Answer from the drawing. Dimensions are ordinates in mm from the lowest x, y and z of the part. Give positions to 0.01 mm unless a question says otherwise; leave off trailing zeros. Order: outer loops, then holes, each group sorted by start corner. A loop starts at its lowest first (then second) coordinate and runs counter-clockwise, first axis right, second up. Notation, with made-up numbers: (34.25, 24.25) - (93.25, 24.25) arc R19 cw to (93.25, 60.25) - close; hole circle Ø7 at (61, 35). An arc over 180 degrees is marked (long way). Write each question's results on one line, items separated by ' | '.
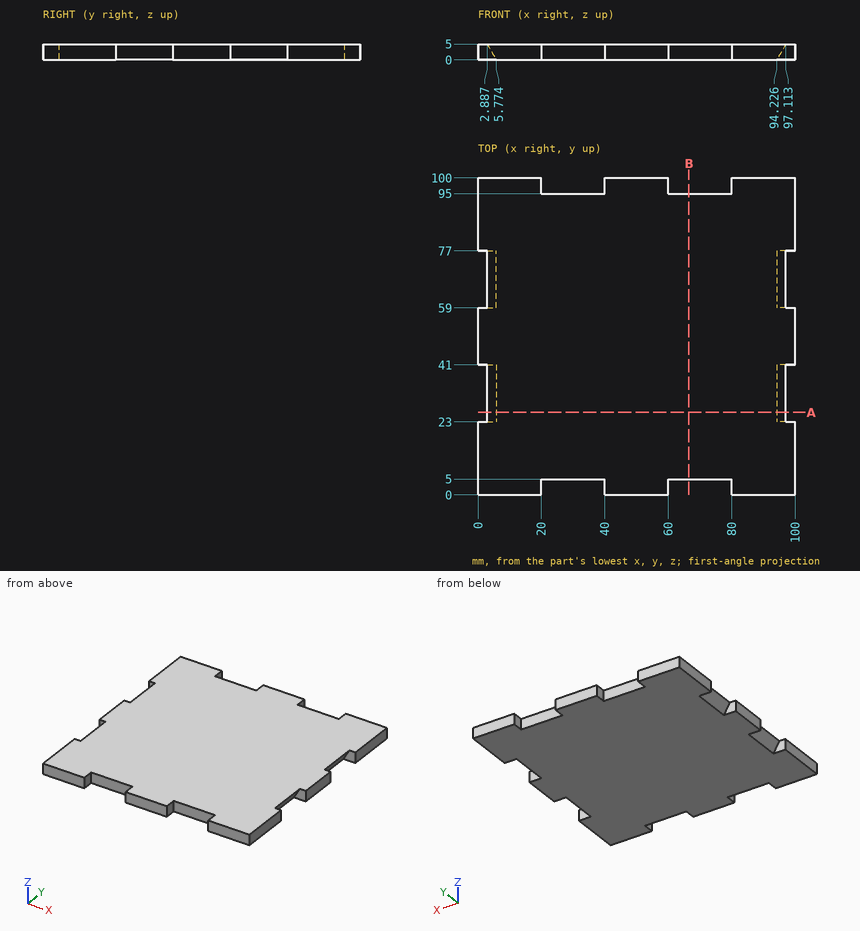
(1) Section A-A (y = 26) is taken. Give the vertices of the cut face in (x, z).
Conclusion:
outline: (2.89, 5) - (5.77, 0) - (94.23, 0) - (97.11, 5) - close
(2) Each of these flat-tipped pins is pushed along its axis until it touches: pin 1 (2 mm diameter, centred on x = 27.5, z = 2, fed in from +Y); pin 2 (2.5 mm diameter, centred on x = 31, z = 3, fed in from -Y). Where does it stop, or does it pass through?
Conclusion:
pin 1: y = 95 | pin 2: y = 5
(3) Section B-B (x = 66.5) is taken. Give the vertices of the cut face in (y, z), plus the area to 3 significant figures.
Conclusion:
outline: (5, 0) - (95, 0) - (95, 5) - (5, 5) - close | area: 450 mm^2
(4) Consider probe 1 along X at (y, z) = (75, 1.3) (1 decimal); probe 2 along X at (y, z) = (25.5, 3.7). Determine where each line is inside the solid, lowest interval first. Write a range as [from, to].
Conclusion:
probe 1: [5, 95] | probe 2: [3.64, 96.36]
